```python
from build123d import *

# Parameters (mm, degrees)
F1_DEPTH = 30
F2_DEPTH = 28.4
F0_W     = 2.5
F0_H     = 3.4
F0_W_2   = 3
F0_W_3   = 7
F0_W_4   = 35.5
F0_W_5   = 70
F3_DEPTH = 17
F0_R     = 1.75
F4_DEPTH = 3
F6_DEPTH = 25
F7_R     = 1.5
F7_W     = 70
F7_H     = 13.8912867606
F8_DEPTH = 25


# Not quite as in the source:
# - ends of sketch curves that miss each other by under 0.0002 mm in the source are joined


with BuildPart() as f1:
    # F0 (on Front) → F1 (new body)
    with BuildSketch(Plane.XZ):
        with BuildLine():
            Line((-180.478038, -29.2658), (-180.478038, -72.7658))
            Line((-180.478038, -72.7658), (-178.478038, -72.7658))
            Line((-178.478038, -72.7658), (-178.478038, -29.2658))
            ThreePointArc((-178.478038, -29.2658), (-177.5993583436, -27.1444796564), (-175.478038, -26.2658))
            Line((-175.478038, -26.2658), (8.521962, -26.2658))
            ThreePointArc((8.521962, -26.2658), (10.6432823436, -27.1444796564), (11.521962, -29.2658))
            Line((11.521962, -29.2658), (11.521962, -71.1658))
            Line((11.521962, -71.1658), (11.521962, -72.7658))
            Line((11.521962, -72.7658), (13.521962, -72.7658))
            Line((13.521962, -72.7658), (13.521962, -29.2658))
            ThreePointArc((13.521962, -29.2658), (12.0574959059, -25.7302660941), (8.521962, -24.2658))
            Line((8.521962, -24.2658), (-175.478038, -24.2658))
            ThreePointArc((-175.478038, -24.2658), (-179.0135719059, -25.7302660941), (-180.478038, -29.2658))
        make_face()
    extrude(amount=F1_DEPTH)

    # F0 (on Front) → F2 (join)
    with BuildSketch(Plane.XZ):
        with BuildLine():
            Line((-178.478038, -29.2658), (-178.478038, -72.7658))
            Line((-178.478038, -72.7658), (-177.478038, -72.7658))
            Line((-177.478038, -72.7658), (-177.478038, -67.7658000352))
            Line((-177.478038, -67.7658000352), (-177.478038, -32.2658))
            ThreePointArc((-177.478038, -32.2658), (-176.0135719059, -28.7302660941), (-172.478038, -27.2658))
            Line((-172.478038, -27.2658), (5.521962, -27.2658))
            ThreePointArc((5.521962, -27.2658), (9.0574959059, -28.7302660941), (10.521962, -32.2658))
            Line((10.521962, -32.2658), (10.521962, -62.7658))
            Line((10.521962, -62.7658), (10.521962, -71.1658))
            Line((10.521962, -71.1658), (11.521962, -71.1658))
            Line((11.521962, -71.1658), (11.521962, -29.2658))
            ThreePointArc((11.521962, -29.2658), (10.6432823436, -27.1444796564), (8.521962, -26.2658))
            Line((8.521962, -26.2658), (-175.478038, -26.2658))
            ThreePointArc((-175.478038, -26.2658), (-177.5993583436, -27.1444796564), (-178.478038, -29.2658))
        make_face()
    extrude(amount=F2_DEPTH)

    # F0 (on Front) → F3 (join)
    with BuildSketch(Plane.XZ):
        with Locations((-168.228038, -69.4658)):
            Rectangle(F0_W, F0_H)
        with Locations((-165.478038, -69.4658)):
            Rectangle(F0_W_2, F0_H)
        with Locations((-160.478038, -69.4658)):
            Rectangle(F0_W_3, F0_H)
        with Locations((-155.478038, -69.4658)):
            Rectangle(F0_W_2, F0_H)
        with Locations((-136.228038, -69.4658)):
            Rectangle(F0_W_4, F0_H)
        with Locations((-83.478038, -69.4658)):
            Rectangle(F0_W_5, F0_H)
        with Locations((-30.728038, -69.4658)):
            Rectangle(F0_W_4, F0_H)
        with Locations((-11.478038, -69.4658)):
            Rectangle(F0_W_2, F0_H)
        with Locations((-6.478038, -69.4658)):
            Rectangle(F0_W_3, F0_H)
        with Locations((-1.478038, -69.4658)):
            Rectangle(F0_W_2, F0_H)
        with BuildLine():
            Line((0.021962, -71.1658), (10.521962, -71.1658))
            Line((10.521962, -71.1658), (10.521962, -62.7658))
            ThreePointArc((10.521962, -62.7658), (9.0574959059, -66.3013339059), (5.521962, -67.7658))
            Line((5.521962, -67.7658), (0.021962, -67.7658))
            Line((0.021962, -67.7658), (0.021962, -71.1658))
        make_face()
    extrude(amount=F3_DEPTH)

    # F0 (on Front) → F4 (join)
    with BuildSketch(Plane.XZ):
        Polygon((-166.978038, -71.1658), (-169.478038, -71.1658), (-169.478038, -72.7658), (11.521962, -72.7658), (11.521962, -71.1658), (10.521962, -71.1658), (0.021962, -71.1658), (-2.978038, -71.1658), (-9.978038, -71.1658), (-12.978038, -71.1658), (-48.478038, -71.1658), (-118.478038, -71.1658), (-153.978038, -71.1658), (-156.978038, -71.1658), (-163.978038, -71.1658), align=None)
        with BuildLine():
            Line((-177.478038, -32.2658), (-177.478038, -67.7658000352))
            ThreePointArc((-177.478038, -67.7658000352), (-173.478038, -64.726809), (-169.4780381264, -67.7658000352))
            Line((-169.4780381264, -67.7658000352), (-166.978038, -67.7658))
            Line((-166.978038, -67.7658), (-163.978038, -67.7658))
            Line((-163.978038, -67.7658), (-156.978038, -67.7658))
            Line((-156.978038, -67.7658), (-153.978038, -67.7658))
            Line((-153.978038, -67.7658), (-118.478038, -67.7658))
            Line((-118.478038, -67.7658), (-48.478038, -67.7658))
            Line((-48.478038, -67.7658), (-12.978038, -67.7658))
            Line((-12.978038, -67.7658), (-9.978038, -67.7658))
            Line((-9.978038, -67.7658), (-2.978038, -67.7658))
            Line((-2.978038, -67.7658), (0.021962, -67.7658))
            Line((0.021962, -67.7658), (5.521962, -67.7658))
            ThreePointArc((5.521962, -67.7658), (9.0574959059, -66.3013339059), (10.521962, -62.7658))
            Line((10.521962, -62.7658), (10.521962, -32.2658))
            ThreePointArc((10.521962, -32.2658), (9.0574959059, -28.7302660941), (5.521962, -27.2658))
            Line((5.521962, -27.2658), (-172.478038, -27.2658))
            ThreePointArc((-172.478038, -27.2658), (-176.0135719059, -28.7302660941), (-177.478038, -32.2658))
        make_face()
        with Locations((-66.878038, -40.4658)):
            Circle(F0_R, mode=Mode.SUBTRACT)
    extrude(amount=F4_DEPTH)

    # F7 (on offset) → F8 (cut)
    with BuildSketch(Plane.XY.offset(-75)):
        with Locations((-11.478038, -9)):
            Circle(F7_R)
        with Locations((-5.478038, -6)):
            Circle(F7_R)
        with Locations((-83.478038, -15.9456433803)):
            Rectangle(F7_W, F7_H)
        with Locations((-161.478038, -6)):
            Circle(F7_R)
        with Locations((-155.478038, -9)):
            Circle(F7_R)
    extrude(amount=F8_DEPTH, mode=Mode.SUBTRACT)


with BuildPart() as f6:
    # F0 (on Front) → F6 (new body)
    with BuildSketch(Plane.XZ):
        Polygon((-177.478038, 13.4356050125), (-177.478038, 12.671673), (-169.478038, 12.671673), (-169.478038, 27.071673), (-118.478038, 27.071673), (-118.478038, 19.571673), (-48.478038, 19.571673), (-48.478038, 27.071673), (10.521962, 27.071673), (10.521962, 38.071673), (-177.478038, 38.071673), (-177.478038, 33.071673), align=None)
    extrude(amount=F6_DEPTH)


solid = f1.part
```
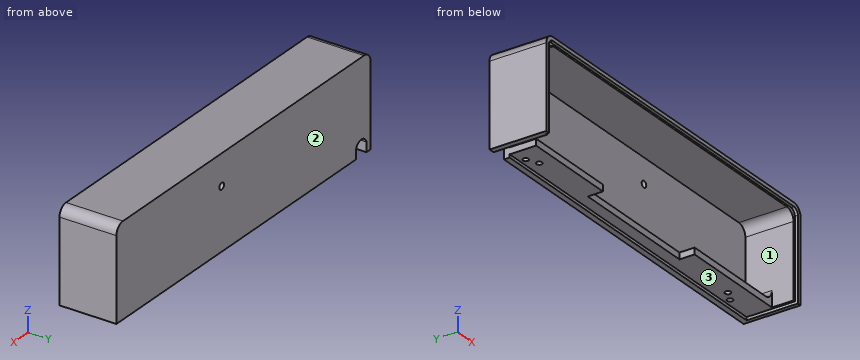
Input: part model. Units: mm. Frame: model coordinates. Face numbers are marked on the shaded views. A direction names the side the tool comes from. Coordinates: 2 decimals unless noted, no trailing zeros. Loops run counter-clockwise (first coordinate to the right, second up) from the corner with the lowest first, then second, coordinate; pieces in that order, holes last. Notation, with made-up numbers: M -33.5,42 L -21.5,42 A17 cw -21.5,60 Z; hole C -39.5,76.25 d9. An arc over 180 degrees is marked long. Use a Markdown table: item, result. Add a question column.
1) Section A-A, the plane z = -46.5. Return the cut outline in (x, y), plus the area to 3 significant figures.
2) Set-up query: the marked faces 1, 2 and 3. Return all of +Z, -Z, +X, -X, +Y, -Y with unobstructed straight access to the full face (end or side cutting, diameter ignored); none if empty.
3) Section B-B, the plane x = -91.5. Return the cut outline in (y, z).
4) Pin query (flat end, axial travel): P1, Ø8, axis at x = -124, z = -48.5, coming from the -Y side; P2, Ø4, axis at x = -29, z = -66, coming from the -Y side; P3, Ø3.5, axis at x = -67.5, z = -68.5, coming from the -Y side. Return the tip coordinate at first contact, or that it passes through.
5) Line query: L1, parallel to X at y = -6, z = -68.7; L2, parallel to X at y = -13, z = -69; L3, parallel to Z at x = 3, y = -14.5. Output: solid intervals per line, ascending. Write a range as from..to.
Answer below:
| question | item | result |
|---|---|---|
| 1 | outline | M -180.48,-30 L -178.48,-30 L -178.48,-28.4 L -177.48,-28.4 L -177.48,-3 L 10.52,-3 L 10.52,-28.4 L 11.52,-28.4 L 11.52,-30 L 13.52,-30 L 13.52,0 L -180.48,0 Z |
| 1 | area | 741 mm2 |
| 2 | face 1 | -Y |
| 2 | face 2 | +Z, -Z, +X, -X, +Y |
| 2 | face 3 | -Z, -Y |
| 3 | outline | M -30,-26.27 L -28.4,-26.27 L -28.4,-27.27 L -3,-27.27 L -3,-67.77 L -9,-67.77 L -9,-71.17 L -3,-71.17 L -3,-72.77 L 0,-72.77 L 0,-24.27 L -30,-24.27 Z |
| 4 | P1 | y = -3 |
| 4 | P2 | y = -17 |
| 4 | P3 | y = -9 |
| 5 | L1 | -180.48..-177.48, -169.48..-162.98, -159.98..-6.98, -3.98..13.52 |
| 5 | L2 | -180.48..-177.48, -169.48..-118.48, -48.48..13.52 |
| 5 | L3 | -71.17..-67.77, -27.27..-24.27 |
